For this review, take the finished solid that the model builds, in its own axes (mm). Face numbers are marked on the shaded views. A direction names the side the tool comes from. Coordinates: 2 decimals unless noted, no trailing zeros. Write each loop counter-clockwise with the first axis right and the second up, starting at its lowest first coordinate (ties: lowest second). Pieces come first, ordered by that corner, then holes. Notation, with made-up numbers: (44.25, 64.5) -> (77.25, 64.5) arc R17 ccw to (77.25, 88.5) -> close; hole circle Ø2 at (84, -9). An arc over 180 degrees is marked (long way). Put each result on its own line as item: value. Start each with the question number.
Item 1: To check wall thickness, follow L1, parallel to X at y = -10, z = 17; L2, parallel to Y at x = 28, z = 14.25; L3, parallel to Z at x = 26, y = -15. State the ranges of each line that lie inside material, in increasing order.
Item 2: Consider section B-B on x = -9. Give the boundary of the cut face in (y, z).
Item 3: Consider section C-C on y = -21.5. Give the boundary of the cut face in (x, z).
Item 4: Consider section A-A on z = 12. Give the boundary of the cut face in (x, y).
Item 5: The part is to be moulded in two halves that separate along Y. For the marked faces 1, 2, 3 and 4, say which applies: +Y half, -Y half, draft (parallel to the pull), parting line (faces both ways), or undercut.
Item 6: Insertion check: P1, Ø5, axis at x = -11.5, y = -6, coming from the -Z side. The pin has a flat end and moves straight along its axis. Give the tip position at first contact, or say it passes through.
Item 7: Consider section D-D on x = 21.5. Give the boundary of the cut face in (y, z), and give its area (3 significant figures).
Item 8: For the marked faces 5 and 6, list the 3-axis set-ups (+Z, -Z, +X, -X, +Y, -Y) from which the entire face can be reached by the end or side of a thin tool; tool diameter is ignored.
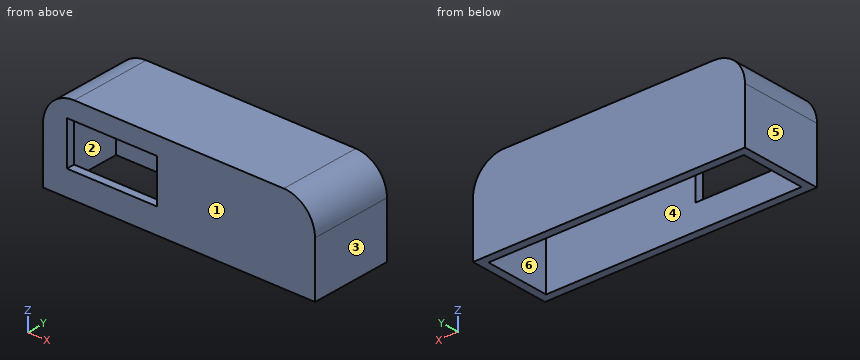
```python
from build123d import *

# Parameters (mm, degrees)
F0_W     = 82.176
F0_H     = 26.12
F1_DEPTH = 25
F2_R     = 9.4154328933
F3_T     = -2.5
F4_W     = 27.2806887515
F4_H     = 13.1527986377
F5_DEPTH = 14.9


# Not quite as in the source:
# - a feature names something its author has since deleted; it is built from what else it names


with BuildPart() as f1:
    # F0 (on Front) → F1 (new body)
    with BuildSketch(Plane.XZ):
        with Locations((10.6781609957, 20.0886886767)):
            Rectangle(F0_W, F0_H)
    extrude(amount=F1_DEPTH)

    # F2
    f2_edges = [f1.edges().sort_by_distance(p)[0] for p in [
        (-30.409839, -12.5, 33.148689),
        (51.766161, -12.5, 33.148689),
    ]]
    fillet(f2_edges, radius=F2_R)

    # F3
    f3_openings = [f1.faces().sort_by_distance(p)[0] for p in [
        (10.678161, -12.5, 7.028689),
    ]]
    offset(amount=F3_T, openings=f3_openings)

    # F4 (on face) → F5 (cut)
    with BuildSketch(Plane.XZ.offset(25)):
        with Locations((-9.543599328, 21.1515771225)):
            Rectangle(F4_W, F4_H)
    extrude(amount=-F5_DEPTH, mode=Mode.SUBTRACT)


solid = f1.part
```
Return value:
1. L1: -30.41 to -27.91, 49.27 to 51.77
1. L2: -25 to -22.5, -2.5 to 0
1. L3: 30.65 to 33.15
2. outline: (-25, 7.03) -> (-22.5, 7.03) -> (-22.5, 14.58) -> (-25, 14.58) -> close; (-25, 27.73) -> (-22.5, 27.73) -> (-22.5, 30.65) -> (-2.5, 30.65) -> (-2.5, 7.03) -> (0, 7.03) -> (0, 33.15) -> (-25, 33.15) -> close
3. outline: (-30.41, 7.03) -> (-27.91, 7.03) -> (-27.91, 23.73) arc R6.92 cw to (-20.99, 30.65) -> (42.35, 30.65) arc R6.92 cw to (49.27, 23.73) -> (49.27, 7.03) -> (51.77, 7.03) -> (51.77, 23.73) arc R9.42 ccw to (42.35, 33.15) -> (-20.99, 33.15) arc R9.42 ccw to (-30.41, 23.73) -> close
4. outline: (-30.41, -25) -> (51.77, -25) -> (51.77, 0) -> (-30.41, 0) -> close; hole (-27.91, -22.5) -> (49.27, -22.5) -> (49.27, -2.5) -> (-27.91, -2.5) -> close
5. face 1: -Y half
5. face 2: undercut
5. face 3: draft
5. face 4: undercut
6. P1: z = 30.65
7. outline: (-25, 7.03) -> (-22.5, 7.03) -> (-22.5, 30.65) -> (-2.5, 30.65) -> (-2.5, 7.03) -> (0, 7.03) -> (0, 33.15) -> (-25, 33.15) -> close
7. area: 181 mm^2
8. face 5: +Z, -Z, -X, +Y, -Y
8. face 6: -Z
